Input: part model. Units: mm. Frame: model coordinates. Face numbers are marked on the shaded views. A direction names the side the tool comes from. Coordinates: 2 decimals unless noted, no trailing zeros. Order: outer loops, then holes, each group sorted by start corner. A loop starts at its lowest first (then second) coordinate and runs counter-clockwise, first axis right, second up. Notation, with made-up numbers: (-33, -17) -> (22, -17) arc R9 cw to (22, 0) -> close; hole circle Ø6 at (24, 82). An arc over 180 degrees is marked (long way). One line per question, with ' | ' between items.
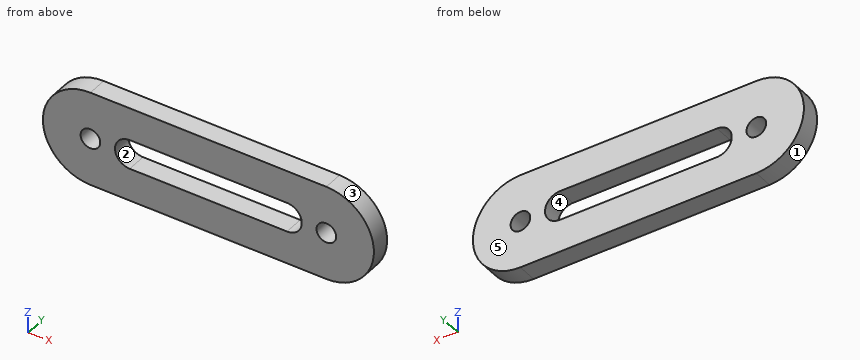
```python
from build123d import *

# Parameters (mm, degrees)
F0_R     = 3.175
F1_DEPTH = 6.35


with BuildPart() as f1:
    # F0 (on Front) → F1 (new body)
    with BuildSketch(Plane.XZ):
        with BuildLine():
            ThreePointArc((38.1, -15.350756), (53.450756, 0), (38.1, 15.350756))
            Line((38.1, 15.350756), (-38.1, 15.350756))
            ThreePointArc((-38.1, 15.350756), (-53.450756, 0), (-38.1, -15.350756))
            Line((-38.1, -15.350756), (38.1, -15.350756))
        make_face()
        with Locations((-38.1, 0)):
            Circle(F0_R, mode=Mode.SUBTRACT)
        with BuildLine():
            Line((-25.4, 4.7625), (25.4, 4.7625))
            ThreePointArc((25.4, 4.7625), (30.1625, 0), (25.4, -4.7625))
            Line((25.4, -4.7625), (-25.4, -4.7625))
            ThreePointArc((-25.4, -4.7625), (-30.1625, 0), (-25.4, 4.7625))
        make_face(mode=Mode.SUBTRACT)
        with Locations((38.1, 0)):
            Circle(F0_R, mode=Mode.SUBTRACT)
    extrude(amount=F1_DEPTH)


solid = f1.part
```
1. Cut plane A-A, the plane x = -7.5. Return loops of the section in (y, z).
Recorded:
outline: (-6.35, -15.35) -> (0, -15.35) -> (0, -4.76) -> (-6.35, -4.76) -> close; (-6.35, 4.76) -> (0, 4.76) -> (0, 15.35) -> (-6.35, 15.35) -> close
2. Access query for the marked faces 1 and 2. Directions: +Z, -Z, +X, -X, +Y, -Y. A direction counts if a zero-diameter tool reaches every point of the face in a straight line with its end or side. Return the directions, or none.
Recorded:
face 1: -X, +Y, -Y | face 2: +Y, -Y
3. Ray query, line 1 (Z direction, x = 38.1, y = -3.75) (3 decimals); line 2 (Z direction, x = -20, y = -1.25); line 3 (X direction, y = -4.5, z = -2). Return the intervals inside material, ascending. Write a range as [from, to].
Recorded:
line 1: z = [-15.351, -3.175], [3.175, 15.351] | line 2: z = [-15.35, -4.76], [4.76, 15.35] | line 3: x = [-53.32, -40.57], [-35.63, -29.72], [29.72, 35.63], [40.57, 53.32]
4. Cut plane D-D, the plane x = -43.5. Return loops of the section in (y, z).
Recorded:
outline: (-6.35, -14.37) -> (0, -14.37) -> (0, 14.37) -> (-6.35, 14.37) -> close
5. Mould query, pull axis Z, two halves, no side actions, for the marked faces 3, 4 and 5. Classes: released by +Z, released by -Z, zero draft, split by the parting line, or undercut.
Recorded:
face 3: split by the parting line | face 4: undercut | face 5: zero draft
6. Cut plane B-B, the plane z = 0. State how many separate pieces and enclosed holes the cut face has, and give its area (3 significant figures).
Recorded:
separate pieces: 4 | enclosed holes: 0 | area: 215 mm^2
